```python
from build123d import *

# Parameters (mm, degrees)
PUSHER_BASE_DEPTH = 15
SKETCH3_R         = 1.95
SCREW_HOLE_DEPTH  = 7.5
SKETCH6_W         = 7.5
SKETCH6_H         = 30.25
PUSHER_HEAD_DEPTH = 3.75
FILLET1_R         = 2


with BuildPart() as part:
    # Sketch1 → pusher base (new body)
    with BuildSketch(Plane.XY):
        Polygon((59.166899441, -45.877477752), (51.666899441, -45.877477752), (44.666899441, -45.877477752), (37.166899441, -45.877477752), (37.166899441, -69.377477752), (41.916899441, -69.377477752), (41.916899441, -64.127477752), (54.416899441, -64.127477752), (54.416899441, -69.377477752), (59.166899441, -69.377477752), align=None)
        with BuildLine():
            Line((48.279417247, -51.877477752), (48.054381634, -51.877477752))
            ThreePointArc((48.054381634, -51.877477752), (39.166899441, -50.877477752), (48.054381634, -49.877477752))
            Line((48.054381634, -49.877477752), (48.279417247, -49.877477752))
            ThreePointArc((48.279417247, -49.877477752), (57.166899441, -50.877477752), (48.279417247, -51.877477752))
        make_face(mode=Mode.SUBTRACT)
    extrude(amount=PUSHER_BASE_DEPTH)

    # Sketch3 → screw hole (cut)
    with BuildSketch(Plane.XZ.offset(64.127477752)):
        with Locations(Location((48.166899441, 7.5, 0), (0, 0, 270))):
            Circle(SKETCH3_R)
    extrude(amount=-SCREW_HOLE_DEPTH, mode=Mode.SUBTRACT)

    # Sketch6 → pusher head (add, symmetric)
    with BuildSketch(Plane.XY.offset(7.5)):
        with Locations((48.166899441, -30.752477752)):
            Rectangle(SKETCH6_W, SKETCH6_H)
    extrude(amount=PUSHER_HEAD_DEPTH, both=True)

    # Fillet1
    # the kernel refuses this fillet: 2 mm, written as the material it takes off along each edge
    with BuildSketch(Plane(origin=(64.166899441, -45.877477752, 0), x_dir=(0, -1, 0), z_dir=(-1, 0, 0)), Plane(origin=(32.166899441, -45.877477752, 15), x_dir=(0, -1, 0), z_dir=(1, 0, 0))) as fillet1_piece_1:
        with BuildLine():
            CenterArc((FILLET1_R, FILLET1_R), FILLET1_R, 180, 90)
            Line((0, FILLET1_R), (0, 0))
            Line((0, 0), (FILLET1_R, 0))
        make_face()
    extrude(amount=32, mode=Mode.SUBTRACT)


solid = part.part
```
CAD build for the part. Positions are in the model's coordinates, mm. A direction names the side the tool comes from. Round coordinates to 2 decimals unless told otherwise and drop trailing zeros. Write each loop counter-clockwise with the first axis right and the second up, starting at its lowest first coordinate (ties: lowest second). Pieces come first, ordered by that corner, then holes.
Item 1: Band-saw the part on C-C on x = 52.75. Write the cut outline in (y, z).
Filled in:
outline: (-64.13, 0) - (-55.38, 0) - (-55.38, 15) - (-64.13, 15) - close; (-46.38, 0.68) arc R2 ccw to (-45.88, 2) - (-45.88, 13) arc R2 ccw to (-46.38, 14.32) - close
Item 2: Mould opens along X. For faces 4 (the cylindrical face through (57.163, -50.694, 7.395)), 5 (the cylindrical face through (46.263, -60.43, 7.923)), 6 (the flat face through (48, -61, 15)), 7 (the flat face through (59.167, -58, 7)) say: released by +X, released by -X, zero draft, split by the parting line, or undercut.
Filled in:
face 4: undercut
face 5: undercut
face 6: zero draft
face 7: released by +X
Item 3: Band-saw the part on D-D on z = 7.5. Write the cut outline in (x, y), then the cut area to 3 significant figures.
Filled in:
outline: (37.17, -69.38) - (41.92, -69.38) - (41.92, -64.13) - (46.22, -64.13) - (46.22, -56.63) - (50.12, -56.63) - (50.12, -64.13) - (54.42, -64.13) - (54.42, -69.38) - (59.17, -69.38) - (59.17, -45.88) - (51.92, -45.88) - (51.92, -15.63) - (44.42, -15.63) - (44.42, -45.88) - (37.17, -45.88) - close; hole (48.05, -51.88) - (48.28, -51.88) arc R4.5 ccw (long way) to (48.28, -49.88) - (48.05, -49.88) arc R4.5 ccw (long way) to start
area: 522 mm2
Item 4: Drill centre lines: L1, parallel to X at y = -61, z = 7.5; L2, parallel to X at y = -54, z = 9; L3, parallel to Y at x = 47.5, z = 3. Where is each one in solid material? Low to high.
Filled in:
L1: x = 37.17 to 46.22, 50.12 to 59.17
L2: x = 37.17 to 40.43, 46.91 to 49.43, 55.91 to 59.17
L3: y = -64.13 to -53.23, -48.52 to -45.88
Item 5: Band-saw the part on B-B on y = -54.5. Write the cut outline in (x, z).
Filled in:
outline: (37.17, 0) - (41, 0) - (41, 15) - (37.17, 15) - close; (46.34, 0) - (50, 0) - (50, 15) - (46.34, 15) - close; (55.34, 0) - (59.17, 0) - (59.17, 15) - (55.34, 15) - close
Item 6: Drop flat-ended pins along their axis: pin 1 Ø7 at (x, y) = (43.67, -50.88) entering from -Z; pin 2 Ø6 at (x, y) = (49, -27) entering from -Z; pin 3 Ø4 at (x, y) = (47.5, -33) entering from +Z; pin 4 Ø8 at (y, z) = (-34, 7.5) entering from -X. Give the stop position or say it passes through.
Filled in:
pin 1: passes through
pin 2: stops at z = 3.75
pin 3: stops at z = 11.25
pin 4: stops at x = 44.42
Item 7: Tool access for faces 1 (the flat face through (48, -31, 3.75)), 2 (the flat face through (49.5, -64.127, 5.7)), 3 (the flat face through (44.417, -31, 8)): list every direction of +Z, -Z, +X, -X, +Y, -Y with a clear straight run to the whole face (end or side of a thin tool).
Filled in:
face 1: -Z, +X, -X, +Y
face 2: +Z, -Z, -Y
face 3: +Z, -Z, -X, +Y
Item 8: Band-saw the part on A-A on z = 4.25. Write the cut outline in (x, y), then the cut area to 3 significant figures.
Filled in:
outline: (37.17, -69.38) - (41.92, -69.38) - (41.92, -64.13) - (54.42, -64.13) - (54.42, -69.38) - (59.17, -69.38) - (59.17, -45.88) - (51.92, -45.88) - (51.92, -15.63) - (44.42, -15.63) - (44.42, -45.88) - (37.17, -45.88) - close; hole (48.05, -51.88) - (48.28, -51.88) arc R4.5 ccw (long way) to (48.28, -49.88) - (48.05, -49.88) arc R4.5 ccw (long way) to start
area: 551 mm2
